Here's how the part is built. I have some questions about the finished solid (model axes, mm). A direction names the side the tool comes from. Give positions to 0.01 mm unless a question says otherwise; leave off trailing zeros. Loops run counter-clockwise (first coordinate to the right, second up) from the corner with the lowest first, then second, coordinate; pieces in that order, holes last. Notation, with made-up numbers: M 68.25,73.25 L 93.25,73.25 A16 ccw 93.25,82.25 Z; hole C 13.25,79 d9. An arc over 180 degrees is marked long. Answer as CSV lines item,"result". Start each with the question number.
Item 1: I want a section at D-D on z = 0. List the corners of the cut face in (x, y) for me, plus the area to 3 significant figures.
Item 2: I want a section at A-A on z = 8. List the corners of the cut face in (x, y) for me, plus the area to 3 significant figures.
Item 3: If we mould it in two halves opening along Z, with no side actions, what happens to faces 1 (the cylindrical face through (-0.027, 0.035, 2.565)), 2 (the flat face through (2, -2.5, 0)), 3 (the cylindrical face through (-2.17, 0.04, 9.76))? For each: released by +Z, released by -Z, zero draft, split by the parting line, or undercut.
Item 4: Will these pins go through, and if not, where does the flat tip stop? P1, Ø3.5, axis at x = -7, z = 0, coming from the +Y side; P2, Ø3, axis at y = -1.5, z = -4, coming from the -X side; P3, Ø2, axis at x = 7.5, y = 0, coming from the +Z side; P4, Ø2.5, axis at x = 0, z = 7, coming from the -Y side.
Item 5: I want a section at B-B on x = 0. List the corners of the cut face in (y, z) for me (3 decimals), plus the area to 4 significant figures.
Item 6: If I drill on line 1 along X through (y, z) = (-0.3, 0); line 2 along Z through (x, y) = (0, -1.3) (3 decimals); line 3 along Z through (x, y) = (1.25, 2.05), over which ranges is the centre line in solid material (lowest first)? Write a range as from..to.
Item 7: I want a section at C-C on x = 8. List the corners of the cut face in (y, z) for me.
Item 8: For faces 4 (the flat face through (-1.758, 0, 0)), 5 (the flat face through (2, 2.5, 0)), which set-ups out of +Z, -Z, +X, -X, +Y, -Y let a thin tool reach every point of the face, with its end or its side?
from build123d import *

# Parameters (mm, degrees)
SKETCH_1_R      = 10
SKETCH_1_R_2    = 1.45
EXTRUDE_1_DEPTH = 2.5


with BuildPart() as part:
    # 草图1 → 凸台-拉伸1 (new body, symmetric)
    with BuildSketch(Plane(origin=(0, 0, 0), x_dir=(1, 0, 0), z_dir=(0, 1, 0))):
        Circle(SKETCH_1_R)
        with Locations((7, 0)):
            Circle(SKETCH_1_R_2, mode=Mode.SUBTRACT)
        with Locations((0, 7)):
            Circle(SKETCH_1_R_2, mode=Mode.SUBTRACT)
        with Locations((-7, 0)):
            Circle(SKETCH_1_R_2, mode=Mode.SUBTRACT)
        with Locations((0, -7)):
            Circle(SKETCH_1_R_2, mode=Mode.SUBTRACT)
        with BuildLine():
            Line((1.7575, 0), (1.7575, 1.868266242))
            ThreePointArc((1.7575, 1.868266242), (0, 2.565), (-1.7575, 1.868266242))
            Line((-1.7575, 1.868266242), (-1.7575, 0))
            Line((-1.7575, 0), (-1.7575, -1.868266242))
            ThreePointArc((-1.7575, -1.868266242), (0, -2.565), (1.7575, -1.868266242))
            Line((1.7575, -1.868266242), (1.7575, 0))
        make_face(mode=Mode.SUBTRACT)
    extrude(amount=EXTRUDE_1_DEPTH, both=True)


solid = part.part
Result:
1,outline,"M -10,-2.5 L -8.45,-2.5 L -8.45,2.5 L -10,2.5 Z; M -5.55,-2.5 L -1.76,-2.5 L -1.76,2.5 L -5.55,2.5 Z; M 1.76,-2.5 L 5.55,-2.5 L 5.55,2.5 L 1.76,2.5 Z; M 8.45,-2.5 L 10,-2.5 L 10,2.5 L 8.45,2.5 Z"
1,area,"53.4 mm^2"
2,outline,"M -6,-2.5 L -1.05,-2.5 L -1.05,2.5 L -6,2.5 Z; M 1.05,-2.5 L 6,-2.5 L 6,2.5 L 1.05,2.5 Z"
2,area,"49.5 mm^2"
3,face 1,"undercut"
3,face 2,"zero draft"
3,face 3,"split by the parting line"
4,P1,"y = 2.5"
4,P2,"x = -9.68"
4,P3,"z = 7.6"
4,P4,"through"
5,outline,"M -2.5,-10 L 2.5,-10 L 2.5,-8.45 L -2.5,-8.45 Z; M -2.5,-5.55 L 2.5,-5.55 L 2.5,-2.565 L -2.5,-2.565 Z; M -2.5,2.565 L 2.5,2.565 L 2.5,5.55 L -2.5,5.55 Z; M -2.5,8.45 L 2.5,8.45 L 2.5,10 L -2.5,10 Z"
5,area,"45.35 mm^2"
6,line 1,"-10..-8.45, -5.55..-1.76, 1.76..5.55, 8.45..10"
6,line 2,"-10..-8.45, -5.55..-2.565, 2.565..5.55, 8.45..10"
6,line 3,"-9.92..-7.73, -6.27..-2.24, 2.24..6.27, 7.73..9.92"
7,outline,"M -2.5,-6 L 2.5,-6 L 2.5,-1.05 L -2.5,-1.05 Z; M -2.5,1.05 L 2.5,1.05 L 2.5,6 L -2.5,6 Z"
8,face 4,"+Y, -Y"
8,face 5,"+Z, -Z, +X, -X, +Y"
